Read the model definition and answer for the solid it produces. Units are mm, in the model's axes. Round coordinates to 2 decimals unless told otherwise and drop trailing zeros. Loops run counter-clockwise (first coordinate to the right, second up) from the corner with the lowest first, then second, coordinate; pieces in that order, holes last. Notation, with made-up numbers: (-12.5, 69) - (29.5, 69) arc R31 ccw to (29.5, 100) - close; hole circle Ø2 at (-3, 25). An arc over 180 degrees is marked (long way). Use one line per item in the form item = value. Start each with the question number.
```python
from build123d import *

# Parameters (mm, degrees)
SKETCH_1_W      = 200
SKETCH_1_H      = 15
EXTRUDE_1_DEPTH = 1
SKETCH_2_W      = 200
SKETCH_2_H      = 1
EXTRUDE_2_DEPTH = 14
M5X0_8_1_D      = 4.2
M3X0_5_1_D      = 2.5
M3X0_5_2_D      = 2.5


with BuildPart() as part:
    # ｽｹｯﾁ1 → ﾎﾞｽ - 押し出し1 (new body)
    with BuildSketch(Plane.XY):
        with Locations((100, 7.5)):
            Rectangle(SKETCH_1_W, SKETCH_1_H)
    extrude(amount=EXTRUDE_1_DEPTH)

    # ｽｹｯﾁ2 → ﾎﾞｽ - 押し出し2 (add)
    with BuildSketch(Plane.XY.offset(1)):
        with Locations((100, 0.5)):
            Rectangle(SKETCH_2_W, SKETCH_2_H)
    extrude(amount=EXTRUDE_2_DEPTH)

    # M5x0.8 ねじ穴1 (through all)
    with Locations(Plane(origin=(0, 0, 0), x_dir=(-1, 0, 0), z_dir=(0, 0, -1))):
        with Locations((-10, 8), (-160, 8)):
            Hole(M5X0_8_1_D / 2)

    # M3x0.5 ねじ穴1 (through all)
    with Locations(Plane(origin=(0, 0, 0), x_dir=(-1, 0, 0), z_dir=(0, -1, 0))):
        with Locations((-193, -7)):
            m3x0_5_1 = Hole(M3X0_5_1_D / 2)

    # M3x0.5 ねじ穴2 (through all)
    with Locations(Plane(origin=(0, 1, 0), x_dir=(1, 0, 0), z_dir=(0, 1, 0))):
        with Locations((80, -8)):
            Hole(M3X0_5_2_D / 2)

    # ﾐﾗｰ2: M3x0.5 ねじ穴1 across plane
    add(m3x0_5_1.mirror(Plane(origin=(100, 0, 0), x_dir=(0, 0, 1), z_dir=(1, 0, 0))), mode=Mode.SUBTRACT)


solid = part.part
```
1) Determine the mould class of faces 1 (the cylindrical face through (162.003, 8.631, 0.507)), 2 (the cylindrical face through (8.452, 9.419, 0.507)), 3 (the flat face through (99, 1, 8)), 4 (the flat face through (99, 8, 1)) for opening direction Y: +Y half, -Y half, draft (parallel to the pull), parting line (faces both ways), or undercut.
2) Flat-ended cylindrical pins translate along their axes: pin 1 (7 mm diameter, centred on x = 143, y = 7.5, fed in from +Z); pin 2 (5 mm diameter, centred on y = 3, z = 4.5, fed in from -X); pin 3 (3 mm diameter, centred on x = 80, z = 8, fed in from +Y); pin 4 (4 mm diameter, centred on x = 160, y = 8, fed in from +Z). Find the tip coordinate at first contact, or state that the pin passes through.
3) A cutting plane is placed at A-A on x = 10. Write down the section's boundary in (y, z), plus the area to 3 significant figures.
4) A cutting plane is placed at C-C on z = 12. Write down the section's boundary in (x, y).
5) Straight lines are drawn through the part: line 1 (Z direction, x = 7, y = 0.5); line 2 (X direction, y = 0.75, z = 8); line 3 (Y direction, x = 10, z = 0.75). For each, find the intervals that lie inside material, in ascending order. Write a range as from..to.
6) A cutting plane is placed at B-B on x = 132.5. Write down the section's boundary in (y, z), plus the area to 3 significant figures.
Checks:
q1.face_1 = undercut
q1.face_2 = undercut
q1.face_3 = +Y half
q1.face_4 = draft
q2.pin_1 = 1
q2.pin_2 = 0
q2.pin_3 = 1
q2.pin_4 = through
q3.outline = (0, 0) - (5.9, 0) - (5.9, 1) - (1, 1) - (1, 15) - (0, 15) - close; (10.1, 0) - (15, 0) - (15, 1) - (10.1, 1) - close
q3.area = 24.8 mm²
q4.outline = (0, 0) - (200, 0) - (200, 1) - (0, 1) - close
q5.line_1 = 0..5.75, 8.25..15
q5.line_2 = 0..6.25, 7.75..78.75, 81.25..192.25, 193.75..200
q5.line_3 = 0..5.9, 10.1..15
q6.outline = (0, 0) - (15, 0) - (15, 1) - (1, 1) - (1, 15) - (0, 15) - close
q6.area = 29.0 mm²
